from build123d import *

# Parameters (mm, degrees)
SKETCH_1_W          = 39
SKETCH_1_H          = 26
EXTRUDE_1_DEPTH     = 10
SKETCH_2_W          = 35
SKETCH_2_H          = 22
CUT_EXTRUDE_1_DEPTH = 8
EXTRUDE_2_DEPTH     = 3
M2_5X0_451_D        = 2.05
M2_5X0_451_DEPTH    = 4
M2_5X0_451_TIP      = 0.615882135
SKETCH_6_W          = 6
SKETCH_6_H          = 6
EXTRUDE_3_DEPTH     = 8
HOLE_WIZARD_M32_D   = 3.4
CUT_EXTRUDE_2_REACH = 49.927
SKETCH_14_W         = 14
SKETCH_14_H         = 5
SKETCH_15_W         = 14
SKETCH_15_H         = 3
EXTRUDE_4_DEPTH     = 4
FILLET_1_R          = 2
FILLET_2_R          = 3


with BuildPart() as part:
    # Эскиз1 → Бобышка-Вытянуть1 (new body)
    with BuildSketch(Plane(origin=(0, 0, 0), x_dir=(1, 0, 0), z_dir=(0, 1, 0))):
        with Locations((19.5, 13)):
            Rectangle(SKETCH_1_W, SKETCH_1_H)
    extrude(amount=EXTRUDE_1_DEPTH)

    # Эскиз2 → Вырез-Вытянуть1 (cut)
    with BuildSketch(Plane(origin=(0, 10, 0), x_dir=(1, 0, 0), z_dir=(0, 1, 0))):
        with Locations((19.5, 13)):
            Rectangle(SKETCH_2_W, SKETCH_2_H)
    extrude(amount=-CUT_EXTRUDE_1_DEPTH, mode=Mode.SUBTRACT)

    # Эскиз3 → Бобышка-Вытянуть2 (add)
    with BuildSketch(Plane(origin=(0, 2, 0), x_dir=(1, 0, 0), z_dir=(0, 1, 0))):
        with BuildLine():
            Line((14.8, 20.1), (14.8, 24))
            Line((14.8, 24), (19.8, 24))
            Line((19.8, 24), (19.8, 20.1))
            ThreePointArc((19.8, 20.1), (17.3, 17.6), (14.8, 20.1))
        make_face()
        with BuildLine():
            Line((19.8, 2), (19.8, 5.9))
            ThreePointArc((19.8, 5.9), (17.3, 8.4), (14.8, 5.9))
            Line((14.8, 5.9), (14.8, 2))
            Line((14.8, 2), (19.8, 2))
        make_face()
    extrude(amount=EXTRUDE_2_DEPTH)

    # Отверстие обработанное метчиком M2.5x0.451
    with Locations(Plane(origin=(0, 5, 0), x_dir=(1, 0, 0), z_dir=(0, 1, 0))):
        with Locations((17.3, 20.1), (17.3, 5.9)):
            Hole(M2_5X0_451_D / 2, depth=M2_5X0_451_DEPTH)
            with Locations((0, 0, -(M2_5X0_451_DEPTH + M2_5X0_451_TIP / 2))):  # 118° drill point
                Cone(0, M2_5X0_451_D / 2, M2_5X0_451_TIP, mode=Mode.SUBTRACT)

    # Эскиз6 → Бобышка-Вытянуть3 (add, through all)
    with BuildSketch(Plane(origin=(0, 2, 0), x_dir=(1, 0, 0), z_dir=(0, 1, 0))):
        with Locations((3, 3)):
            Rectangle(SKETCH_6_W, SKETCH_6_H)
        with Locations((36, 23)):
            Rectangle(SKETCH_6_W, SKETCH_6_H)
        with Locations((36, 3)):
            Rectangle(SKETCH_6_W, SKETCH_6_H)
        with Locations((3, 23)):
            Rectangle(SKETCH_6_W, SKETCH_6_H)
    extrude(amount=EXTRUDE_3_DEPTH)

    # Отверстие с зазором M32 (through all)
    with Locations(Plane(origin=(0, 10, 0), x_dir=(1, 0, 0), z_dir=(0, 1, 0))):
        with Locations((3, 23), (36, 23), (36, 3), (3, 3)):
            Hole(HOLE_WIZARD_M32_D / 2)

    # Эскиз14 → Вырез-Вытянуть2 (cut, up to next)
    with BuildSketch(Plane(origin=(39, 0, 0), x_dir=(0, 0, -1), z_dir=(1, 0, 0)), mode=Mode.PRIVATE) as cut_extrude_2_sk1:
        with Locations((13, 7.5)):
            Rectangle(SKETCH_14_W, SKETCH_14_H)
    cut_extrude_2_tool1 = extrude(cut_extrude_2_sk1.sketch, amount=-CUT_EXTRUDE_2_REACH, mode=Mode.PRIVATE) & part.part
    add(cut_extrude_2_tool1.solids().sort_by_distance((39, 7.5, -13))[0], mode=Mode.SUBTRACT)

    # Эскиз15 → Бобышка-Вытянуть4 (add)
    with BuildSketch(Plane.ZY.offset(-37)):
        with Locations((-13, 3.5)):
            Rectangle(SKETCH_15_W, SKETCH_15_H)
    extrude(amount=EXTRUDE_4_DEPTH)

    # Скругление1
    fillet_1_edges = [part.edges().sort_by_distance(p)[0] for p in [
        (33, 6, -2),
        (2, 6, -20),
        (6, 6, -24),
        (19.8, 3.5, -24),
        (14.8, 3.5, -24),
        (14.8, 3.5, -2),
        (19.8, 3.5, -2),
        (2, 6, -6),
        (6, 6, -2),
        (33, 6, -24),
    ]]
    fillet(fillet_1_edges, radius=FILLET_1_R)

    # Скругление2
    fillet_2_edges = [part.edges().sort_by_distance(p)[0] for p in [
        (0, 5, -26),
        (39, 5, -26),
        (39, 5, 0),
        (0, 5, 0),
    ]]
    fillet(fillet_2_edges, radius=FILLET_2_R)


solid = part.part
The listing builds one solid part. Answer for the finished solid, in the listing's coordinates (mm). A direction names the side the tool comes from. Round coordinates to 2 decimals unless told otherwise and drop trailing zeros. Write each loop counter-clockwise with the first axis right and the second up, starting at its lowest first coordinate (ties: lowest second). Pieces come first, ordered by that corner, then holes. Notation, with made-up numbers: M -6,5.5 L 27,5.5 A22 ccw 27,33.5 Z; hole C 42,35.25 d11. An arc over 180 degrees is marked long. Write each question's results on one line, items separated by ' | '. Start each with the question number.
Item 1: Find section A-A on y = 8. Give the number of separate pieces and of enclosed holes in the cut face, and give its area (3 significant figures).
Item 2: Given pin 1 Ø1.9 at (x, z) = (15.5, -4) entering from +Y; pin 2 Ø5 at (x, z) = (20.5, -12.5) entering from +Y, each flat-ended and moving along its own axis, determine where each tip first touches the part or whether it passes through.
Item 3: Which of the six approach directions +Z, -Z, +X, -X, +Y, -Y give full straight-line access (tool end or side, diameter ignored) to faces 4 (the flat face through (19, 5, -26)), 5 (the cylindrical face through (2.57, 6.06, -6.6))?
Item 4: Straight lines are drawn through the part: probe 1 along Z at (x, y) = (17.3, 2.55) (3 decimals); probe 2 along X at (y, z) = (3.5, -20.1) (3 decimals); probe 3 along X at (y, z) = (9.5, -20.75). For each, find the intervals that lie inside material, in ascending order.
Item 5: The mould has two halves that part along X. Classify faces 1 (the cylindrical face through (14.2, 3.52, -23.43)), 2 (the flat face through (36, 7, -6)), 3 (the cylindrical face through (38.1, 4.93, -25.14)): +X half, -X half, draft (parallel to the pull), parting line (faces both ways), or undercut.
Item 6: Find section D-D on x = 6.5. Write down the section's boundary in (y, z), and give its area (3 significant figures).
Item 7: Find section B-B on x = 26.5. Write down the section's boundary in (y, z).
Answer block:
1) separate pieces: 1 | enclosed holes: 4 | area: 241 mm²
2) pin 1: stops at y = 5 | pin 2: stops at y = 2
3) face 4: -Z, +X, -X, +Y, -Y | face 5: +Y
4) probe 1: z = -26 to -21.125, -19.075 to -17.6, -8.4 to -6.925, -4.875 to 0 | probe 2: x = 0 to 6, 14.8 to 16.275, 18.325 to 19.8, 33 to 39 | probe 3: x = 0 to 6, 33 to 39
5) face 1: undercut | face 2: draft | face 3: +X half
6) outline: M 0,-26 L 10,-26 L 10,-23.32 L 2,-23.32 L 2,-2.68 L 10,-2.68 L 10,0 L 0,0 Z | area: 94.8 mm²
7) outline: M 0,-26 L 10,-26 L 10,-24 L 2,-24 L 2,-2 L 10,-2 L 10,0 L 0,0 Z
